Can you work these out from the drawing? Everything is in mm from the part's minimum corner. Coordinates: 2 decimals unless noted, no trailing zeros. Order: outer loops, then holes, each group sorted by start corner. A loop starts at its lowest first (then second) coordinate and runs counter-clockwise, first axis right, second up. Notation, with made-up numbers: (33, -27.5) - (80, -27.5) arc R21 cw to (80, -8.5) - close; hole circle Ø9 at (29, -2.5). An arc over 180 degrees is marked (long way). Answer as CSV lines item,"result". Start each with the question number.
Item 1: Imagine slicing it at B-B on z = 416. List the corners of the cut face in (x, y) for me.
Item 2: Imagine slicing it at C-C on z = 275. List the corners of the cut face in (x, y) for me.
Item 3: I need wall thicknesses on line 1 (Z direction, x = 453, y = 12); line 2 (X direction, y = 11.25, z = 35); line 3 (Y direction, x = 504, z = 275). Which ranges of each line are inside material? Lowest first, please.
Item 4: Imagine slicing it at A-A on x = 275. List the corners of the cut face in (y, z) for me, and give its area (3 significant figures).
Item 5: Imagine slicing it at D-D on x = 163.5. List the corners of the cut face in (y, z) for me.
Item 6: I'm going to push flat-ended pins straight in: pin 1 (10 mm diameter, centred on x = 84, y = 21.5, fed in from +Z); pin 2 (1.5 mm diameter, centred on x = 148, y = 11, fed in from -Z); pin 3 (14.5 mm diameter, centred on y = 12.5, z = 275, fed in from +X); pin 4 (10 mm diameter, centred on x = 253, z = 325, fed in from -Y). Where does each tip first touch, or does it pass through?
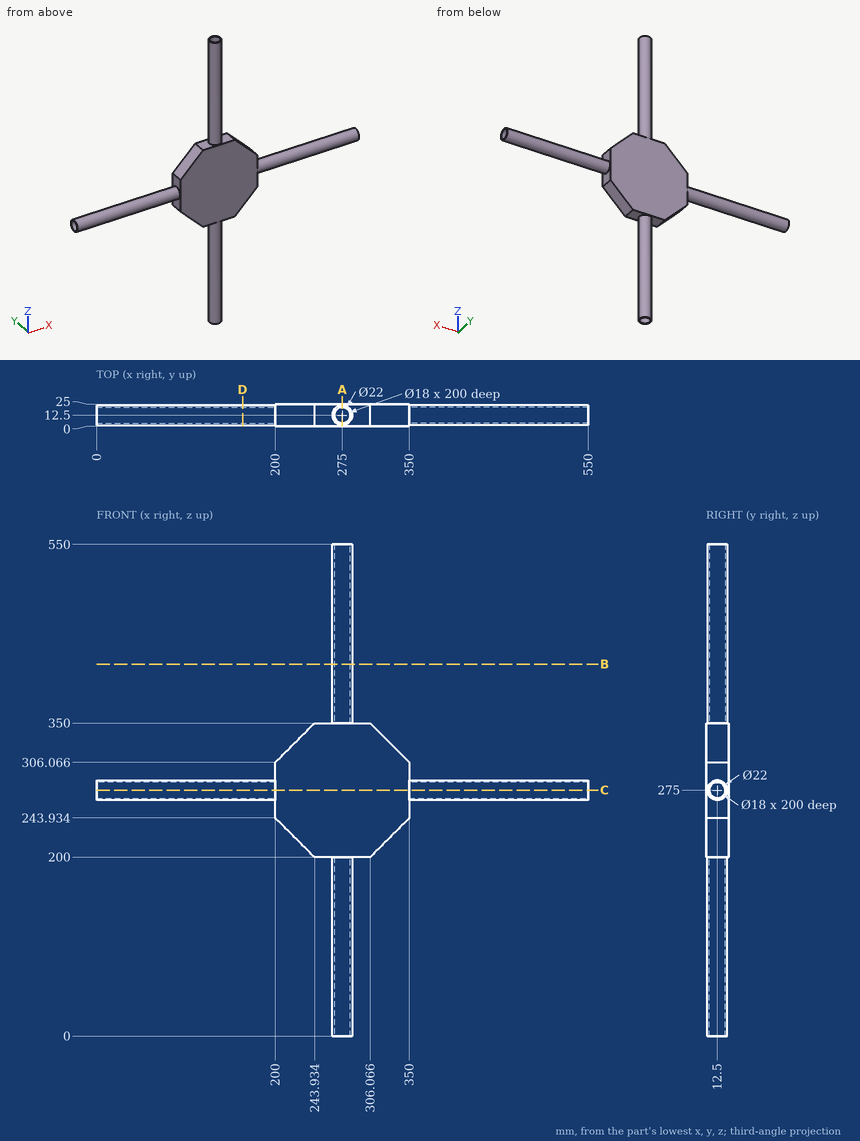
Responses:
1,outline,"circle Ø22 at (275, 12.5); hole circle Ø18 at (275, 12.5)"
2,outline,"(0, 1.5) - (200, 1.5) - (200, 0) - (350, 0) - (350, 1.5) - (550, 1.5) - (550, 3.5) - (350, 3.5) - (350, 21.5) - (550, 21.5) - (550, 23.5) - (350, 23.5) - (350, 25) - (200, 25) - (200, 23.5) - (0, 23.5) - (0, 21.5) - (200, 21.5) - (200, 3.5) - (0, 3.5) - close"
3,line 1,"z = 264.01 to 266.01, 283.99 to 285.99"
3,line 2,"x = 264.07 to 266.09, 283.91 to 285.93"
3,line 3,"y = 1.5 to 3.5, 21.5 to 23.5"
4,outline,"(0, 200) - (1.5, 200) - (1.5, 0) - (3.5, 0) - (3.5, 200) - (21.5, 200) - (21.5, 0) - (23.5, 0) - (23.5, 200) - (25, 200) - (25, 350) - (23.5, 350) - (23.5, 550) - (21.5, 550) - (21.5, 350) - (3.5, 350) - (3.5, 550) - (1.5, 550) - (1.5, 350) - (0, 350) - close"
4,area,"5,350 mm^2"
5,outline,"circle Ø22 at (12.5, 275); hole circle Ø18 at (12.5, 275)"
6,pin 1,"stops at z = 285.25"
6,pin 2,"stops at z = 264.03"
6,pin 3,"stops at x = 350"
6,pin 4,"stops at y = 0"
